```python
from build123d import *

# Parameters (mm, degrees)
SKETCH1_W               = 965.2
SKETCH1_H               = 508
BOSS_EXTRUDE1_DEPTH     = 100
CUT_EXTRUDE1_DEPTH      = 555.453568841
CUT_EXTRUDE1_DEPTH_BACK = 555.453568841
SKETCH2_R               = 12.7


with BuildPart() as part:
    # Sketch1 → Boss-Extrude1 (new body)
    with BuildSketch(Plane.XY):
        Rectangle(SKETCH1_W, SKETCH1_H)
    extrude(amount=-BOSS_EXTRUDE1_DEPTH)

    # Sketch2 → Cut-Extrude1 (cut, two sides: drawn at the far end of the back side and taken through both)
    with BuildSketch(Plane.XY.offset(-CUT_EXTRUDE1_DEPTH_BACK)):
        with Locations((-427.956480022, 0)):
            Circle(SKETCH2_R)
    extrude(amount=CUT_EXTRUDE1_DEPTH + CUT_EXTRUDE1_DEPTH_BACK, mode=Mode.SUBTRACT)


solid = part.part
```
Geometry: final body of the model. Coordinates: model frame, mm. Round coordinates to 2 decimals unless told otherwise and drop trailing zeros. Write each loop counter-clockwise with the first axis right and the second up, starting at its lowest first coordinate (ties: lowest second). Pieces come first, ordered by that corner, then holes.
Item 1: Material intervals for L1, parallel to X at y = 0, z = -56, sorted ascending.
Item 2: Pin query (flat end, axial travel): P1, Ø15, axis at x = -427.96, y = 0, coming from the -Z side. Return the tip coordinate at first contact, or that it passes through.
Item 3: Section query A-A (y = 0). Return loops of the section in (x, z), plus the area to 3 significant figures.
Item 4: Mould query, pull axis X, two halves, no side actions, for faces 1 (the face through (-7, 4, -100)), 2 (the face through (-415.84, 3.81, -50.7)), 3 (the face through (482.6, -4, -49)). Classes: +X half, -X half, draft (parallel to the pull), parting line (faces both ways), or undercut.
Completed:
1. L1: x = -482.6 to -440.66, -415.26 to 482.6
2. P1: passes through
3. outline: (-482.6, -100) - (-440.66, -100) - (-440.66, 0) - (-482.6, 0) - close; (-415.26, -100) - (482.6, -100) - (482.6, 0) - (-415.26, 0) - close
3. area: 94,000 mm2
4. face 1: draft
4. face 2: undercut
4. face 3: +X half
